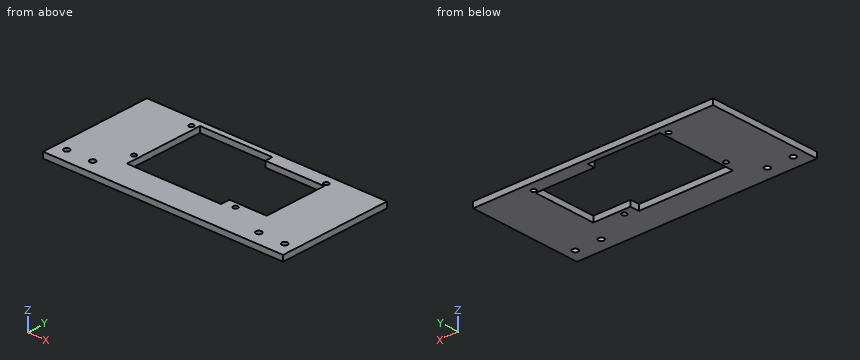
```python
from build123d import *

# Parameters (mm, degrees)
ESQUISSE1_W             = 250
ESQUISSE1_H             = 118.414906094
BOSS_EXTRU_1_DEPTH      = 6
ENL_V_MAT_EXTRU_1_REACH = 231.506
ENL_V_MAT_EXTRU_2_REACH = 231.506
ESQUISSE3_R             = 2.5
ENL_V_MAT_EXTRU_3_REACH = 231.506
ESQUISSE4_R             = 3


with BuildPart() as part:
    # Esquisse1 → Boss.-Extru.1 (new body)
    with BuildSketch(Plane.XY):
        with Locations((75, -53.207453047)):
            Rectangle(ESQUISSE1_W, ESQUISSE1_H)
    extrude(amount=BOSS_EXTRU_1_DEPTH)

    # Esquisse2 → Enl_v. mat.-Extru.1 (cut, up to next)
    with BuildSketch(Plane(origin=(0, 0, 0), x_dir=(-1, 0, 0), z_dir=(0, 0, -1)), mode=Mode.PRIVATE) as enl_v_mat_extru_1_sk1:
        Polygon((-10.782435162, 0), (-10.782435162, -83.25), (-108.778675483, -83.25), (-108.778675483, -73.68186315), (-147.5, -73.68186315), (-147.5, -8), (-86.152674603, -8), (-86.152674603, 0), align=None)
    enl_v_mat_extru_1_tool1 = extrude(enl_v_mat_extru_1_sk1.sketch, amount=-ENL_V_MAT_EXTRU_1_REACH, mode=Mode.PRIVATE) & part.part
    add(enl_v_mat_extru_1_tool1.solids().sort_by_distance((75.657683, -42.082804, 0))[0], mode=Mode.SUBTRACT)

    # Esquisse3 → Enl_v. mat.-Extru.2 (cut, up to next)
    with BuildSketch(Plane(origin=(0, 0, 0), x_dir=(-1, 0, 0), z_dir=(0, 0, -1)), mode=Mode.PRIVATE) as enl_v_mat_extru_2_sk1:
        with Locations((-5.5, -69.5)):
            Circle(ESQUISSE3_R)
    enl_v_mat_extru_2_tool1 = extrude(enl_v_mat_extru_2_sk1.sketch, amount=-ENL_V_MAT_EXTRU_2_REACH, mode=Mode.PRIVATE) & part.part
    # Esquisse3 → Enl_v. mat.-Extru.2 (cut, up to next)
    with BuildSketch(Plane(origin=(0, 0, 0), x_dir=(-1, 0, 0), z_dir=(0, 0, -1)), mode=Mode.PRIVATE) as enl_v_mat_extru_2_sk2:
        with Locations((-5.5, -4)):
            Circle(ESQUISSE3_R)
    enl_v_mat_extru_2_tool2 = extrude(enl_v_mat_extru_2_sk2.sketch, amount=-ENL_V_MAT_EXTRU_2_REACH, mode=Mode.PRIVATE) & part.part
    # Esquisse3 → Enl_v. mat.-Extru.2 (cut, up to next)
    with BuildSketch(Plane(origin=(0, 0, 0), x_dir=(-1, 0, 0), z_dir=(0, 0, -1)), mode=Mode.PRIVATE) as enl_v_mat_extru_2_sk3:
        with Locations((-146, -4)):
            Circle(ESQUISSE3_R)
    enl_v_mat_extru_2_tool3 = extrude(enl_v_mat_extru_2_sk3.sketch, amount=-ENL_V_MAT_EXTRU_2_REACH, mode=Mode.PRIVATE) & part.part
    # Esquisse3 → Enl_v. mat.-Extru.2 (cut, up to next)
    with BuildSketch(Plane(origin=(0, 0, 0), x_dir=(-1, 0, 0), z_dir=(0, 0, -1)), mode=Mode.PRIVATE) as enl_v_mat_extru_2_sk4:
        with Locations((-120.5, -79.5)):
            Circle(ESQUISSE3_R)
    enl_v_mat_extru_2_tool4 = extrude(enl_v_mat_extru_2_sk4.sketch, amount=-ENL_V_MAT_EXTRU_2_REACH, mode=Mode.PRIVATE) & part.part
    add(enl_v_mat_extru_2_tool1.solids().sort_by_distance((5.5, -69.5, 0))[0], mode=Mode.SUBTRACT)
    add(enl_v_mat_extru_2_tool2.solids().sort_by_distance((5.5, -4, 0))[0], mode=Mode.SUBTRACT)
    add(enl_v_mat_extru_2_tool3.solids().sort_by_distance((146, -4, 0))[0], mode=Mode.SUBTRACT)
    add(enl_v_mat_extru_2_tool4.solids().sort_by_distance((120.5, -79.5, 0))[0], mode=Mode.SUBTRACT)

    # Esquisse4 → Enl_v. mat.-Extru.3 (cut, up to next)
    with BuildSketch(Plane(origin=(0, 0, 0), x_dir=(-1, 0, 0), z_dir=(0, 0, -1)), mode=Mode.PRIVATE) as enl_v_mat_extru_3_sk1:
        with Locations((-188.5, -97.914906094)):
            Circle(ESQUISSE4_R)
    enl_v_mat_extru_3_tool1 = extrude(enl_v_mat_extru_3_sk1.sketch, amount=-ENL_V_MAT_EXTRU_3_REACH, mode=Mode.PRIVATE) & part.part
    # Esquisse4 → Enl_v. mat.-Extru.3 (cut, up to next)
    with BuildSketch(Plane(origin=(0, 0, 0), x_dir=(-1, 0, 0), z_dir=(0, 0, -1)), mode=Mode.PRIVATE) as enl_v_mat_extru_3_sk2:
        with Locations((-161.5, -97.914906094)):
            Circle(ESQUISSE4_R)
    enl_v_mat_extru_3_tool2 = extrude(enl_v_mat_extru_3_sk2.sketch, amount=-ENL_V_MAT_EXTRU_3_REACH, mode=Mode.PRIVATE) & part.part
    enl_v_mat_extru_3_1 = enl_v_mat_extru_3_tool1.solids().sort_by_distance((188.5, -97.914906, 0))[0]
    add(enl_v_mat_extru_3_1, mode=Mode.SUBTRACT)
    enl_v_mat_extru_3_2 = enl_v_mat_extru_3_tool2.solids().sort_by_distance((161.5, -97.914906, 0))[0]
    add(enl_v_mat_extru_3_2, mode=Mode.SUBTRACT)
    enl_v_mat_extru_3 = enl_v_mat_extru_3_1 + enl_v_mat_extru_3_2  # Enl_v. mat.-Extru.3 as one shape, for the pattern or mirror that repeats it

    # Sym_trie1: Enl_v. mat.-Extru.3 across plane
    add(enl_v_mat_extru_3.mirror(Plane(origin=(75, 0, 0), x_dir=(0, 0, 1), z_dir=(1, 0, 0))), mode=Mode.SUBTRACT)


solid = part.part
```
Here's how the part is built. I have some questions about the finished solid (model axes, mm). Coordinates: 2 decimals unless noted, no trailing zeros. Write each loop counter-clockwise with the first axis right and the second up, starting at its lowest first coordinate (ties: lowest second). Pieces come first, ordered by that corner, then holes. Notation, with made-up numbers: (12, 62) - (48, 62) arc R4 cw to (48, 68) - close; hole circle Ø5 at (35, -15). An arc over 180 degrees is marked (long way). One line per item, written item: value.
1) Suppose I cut it at C-C on x = 5.5. Write out the boundary of the cut face in (y, z), and give its area (3 significant figures).
Model answer:
outline: (-112.41, 0) - (-72, 0) - (-72, 6) - (-112.41, 6) - close; (-67, 0) - (-6.5, 0) - (-6.5, 6) - (-67, 6) - close; (-1.5, 0) - (6, 0) - (6, 6) - (-1.5, 6) - close
area: 650 mm²
2) Suppose I cut it at A-A on y = -18. Write out the boundary of the cut face in (x, z).
Model answer:
outline: (-50, 0) - (10.78, 0) - (10.78, 6) - (-50, 6) - close; (147.5, 0) - (200, 0) - (200, 6) - (147.5, 6) - close
3) I need wall thicknesses on line 1 along Y through (x, z) = (120.5, 2.6); line 2 along Y through (x, z) = (161.5, 2.4); line 3 along X through (y, z) = (-23.5, 3.9). Which ranges of each line are inside material? Lowest first, please.
Model answer:
line 1: y = -112.41 to -82, -77 to -73.68, -8 to 6
line 2: y = -112.41 to -100.91, -94.91 to 6
line 3: x = -50 to 10.78, 147.5 to 200
4) Suppose I cut it at D-D on y = -79.5. Write out the boundary of the cut face in (x, z).
Model answer:
outline: (-50, 0) - (10.78, 0) - (10.78, 6) - (-50, 6) - close; (108.78, 0) - (118, 0) - (118, 6) - (108.78, 6) - close; (123, 0) - (200, 0) - (200, 6) - (123, 6) - close
5) Suppose I cut it at B-B on x = 139. Write out the boundary of the cut face in (y, z), and give its area (3 significant figures).
Model answer:
outline: (-112.41, 0) - (-73.68, 0) - (-73.68, 6) - (-112.41, 6) - close; (-8, 0) - (6, 0) - (6, 6) - (-8, 6) - close
area: 316 mm²
